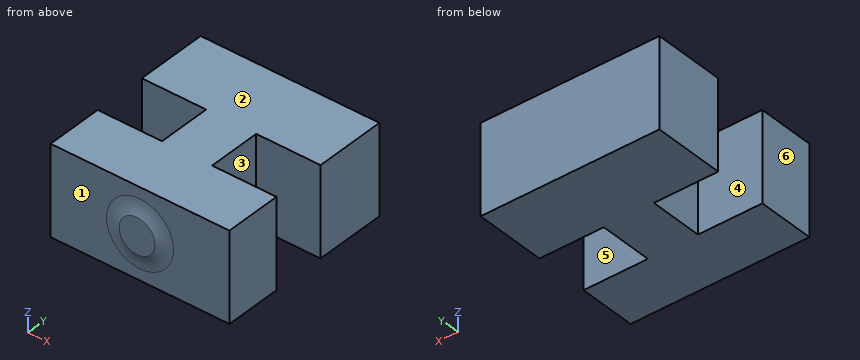
```python
from build123d import *

# Parameters (mm, degrees)
BODY_DEPTH = 6.35
SKETCH4_R  = 1.27
FLAG_DEPTH = 0.254
HOLDER_R   = 2.54


with BuildPart() as part:
    # Sketch2 → body (new body)
    with BuildSketch(Plane.XY):
        Polygon((0, 0), (12.7, 0), (12.7, -5.08), (8.128, -5.08), (8.128, -8.89), (12.7, -8.89), (12.7, -12.954), (0, -12.954), (0, -8.89), (4.572, -8.89), (4.572, -5.08), (0, -5.08), align=None)
    extrude(amount=BODY_DEPTH)

    # Sketch4 → flag (add)
    with BuildSketch(Plane.XZ.offset(12.954)):
        with Locations(Location((6.35, 3.175, 0), (0, 0, 90))):
            Circle(SKETCH4_R)
    extrude(amount=FLAG_DEPTH)

    # holder
    # the kernel refuses this fillet: 2.54 mm, written as the material it adds along each edge
    with BuildSketch(Plane(origin=(6.35, -12.954, 3.175), x_dir=(0, 0, 1), z_dir=(1, 0, 0))) as holder_piece_1:
        with BuildLine():
            CenterArc((2.377160332, 2.54), HOLDER_R, 244.158067237, 25.841932763)
            Line((1.27, 0.254), (1.27, 0))
            Line((1.27, 0), (2.377160332, 0))
        make_face()
    revolve(axis=Axis((6.35, -12.954, 3.175), (0, -1, 0)))


solid = part.part
```
Part model, mm, in its own coordinate system. Face numbers are marked on the shaded views. A direction names the side the tool comes from. Round coordinates to 2 decimals unless told otherwise and drop trailing zeros. Loops run counter-clockwise (first coordinate to the right, second up) from the corner with the lowest first, then second, coordinate; pieces in that order, holes last. Notation, with made-up numbers: (-8.75, 25) -> (23.25, 25) arc R26 ccw to (23.25, 53) -> close; hole circle Ø9 at (79, 51). An arc over 180 degrees is marked (long way). Use one line per item in the form item = value. Start each with the question number.
Item 1: Band-saw the part on A-A (x = 3.25). List the corners of the cut face in (y, z), plus the area to 3 significant figures.
Item 2: Tool access for the marked faces 4, 5 and 6: list every direction of +Z, -Z, +X, -X, +Y, -Y with a clear straight run to the whole face (end or side of a thin tool).
Item 3: Band-saw the part on B-B (z = 0.5). List the corners of the cut face in (x, y), plus the area to 3 significant figures.
Item 4: Drill centre lines: line 1 along Y through (x, z) = (3.25, 2); line 2 along Y through (x, z) = (7.5, 6.25); line 3 along X through (y, z) = (-7.25, 5). Where is each one in solid material? Low to high.
Item 5: Two-plate mould, pull along Y, no slides. Class the marked faces 1, 2 and 3: released by +Y, released by -Y, zero draft, split by the parting line, or undercut.
Item 6: Band-saw the part on C-C (y = -6.5). List the corners of the cut face in (x, z).
Item 7: Drop flat-ended pins along their axis: pin 1 Ø2.5 at (x, z) = (11, 4) entering from -Y; pin 2 Ø2 at (y, z) = (-6.5, 4.5) entering from -X. Give the stop position or say it passes through.
Data:
q1.outline = (-12.95, 0) -> (-8.89, 0) -> (-8.89, 6.35) -> (-12.95, 6.35) -> close; (-5.08, 0) -> (0, 0) -> (0, 6.35) -> (-5.08, 6.35) -> close
q1.area = 58.1 mm^2
q2.face_4 = +Z, -Z, -X
q2.face_5 = +Z, -Z, +X
q2.face_6 = +Z, -Z, -X, +Y, -Y
q3.outline = (0, -12.95) -> (12.7, -12.95) -> (12.7, -8.89) -> (8.13, -8.89) -> (8.13, -5.08) -> (12.7, -5.08) -> (12.7, 0) -> (0, 0) -> (0, -5.08) -> (4.57, -5.08) -> (4.57, -8.89) -> (0, -8.89) -> close
q3.area = 130 mm^2
q4.line_1 = -12.95 to -8.89, -5.08 to 0
q4.line_2 = -12.95 to 0
q4.line_3 = 4.57 to 8.13
q5.face_1 = released by -Y
q5.face_2 = zero draft
q5.face_3 = undercut
q6.outline = (4.57, 0) -> (8.13, 0) -> (8.13, 6.35) -> (4.57, 6.35) -> close
q7.pin_1 = -12.95
q7.pin_2 = 4.57
